Source: CAD feature listing. Evaluate the final solid. Frame: model axes, mm. Face numbers are marked on the shaded views. Round coordinates to 2 decimals unless told otherwise and drop trailing zeros. Write each question's results on one line, items separated by ' | '. Start each with the question number.
1. Draft query along Y for the marked faces 1 and 2. Return one class per face: released by +Y, released by -Y, zero draft, split by the parting line, or undercut.
2. Section A-A on y = 4.25. Give the number of separate pieces and of enclosed holes in the cut face, and give its area (3 significant figures).
3. Ray query, line 1 (X direction, y = 3.25, z = 0); line 2 (X direction, y = 1.75, z = 42) (3 decimals); line 3 (Z direction, x = 1, y = 11). Return the intervals inside material, ascending.
4. Contact query for flat-ended pins moving along their axis: pin 1 Ø6.5 at (y, z) = (9.5, 42.5) entering from +X; pin 2 Ø4 at (y, z) = (9, -42.5) entering from -X. Output: stop coordinate, or through.
from build123d import *

# Parameters (mm, degrees)
SKETCH1_W          = 304.8
SKETCH1_H          = 190.5
EXTRUDE1_DEPTH     = 12.7
SKETCH2_W          = 12.7
SKETCH2_H          = 19.05
EXTRUDE2_DEPTH     = 181.165514181
SKETCH3_R          = 1.5875
CUT_EXTRUDE1_DEPTH = 181.165514181
SKETCH4_R          = 2.032
CUT_EXTRUDE2_DEPTH = 181.165514181


with BuildPart() as part:
    # Sketch1 → Extrude1 (new body)
    with BuildSketch(Plane(origin=(0, 0, 0), x_dir=(1, 0, 0), z_dir=(0, 1, 0))):
        Rectangle(SKETCH1_W, SKETCH1_H)
    extrude(amount=EXTRUDE1_DEPTH)

    # Sketch2 → Extrude2 (cut, through all)
    with BuildSketch(Plane(origin=(0, 12.7, 0), x_dir=(1, 0, 0), z_dir=(0, 1, 0))):
        with Locations((-48.895, 44.45)):
            Rectangle(SKETCH2_W, SKETCH2_H)
        with Locations((48.895, 44.45)):
            Rectangle(SKETCH2_W, SKETCH2_H)
        with Locations((-48.895, -44.45)):
            Rectangle(SKETCH2_W, SKETCH2_H)
        with Locations((48.895, -44.45)):
            Rectangle(SKETCH2_W, SKETCH2_H)
        with Locations((146.05, 44.45)):
            Rectangle(SKETCH2_W, SKETCH2_H)
        with Locations((-146.05, 44.45)):
            Rectangle(SKETCH2_W, SKETCH2_H)
        with Locations((146.05, -44.45)):
            Rectangle(SKETCH2_W, SKETCH2_H)
        with Locations((-146.05, -44.45)):
            Rectangle(SKETCH2_W, SKETCH2_H)
    extrude(amount=-EXTRUDE2_DEPTH, mode=Mode.SUBTRACT)

    # Sketch3 → Cut-Extrude1 (cut, through all)
    with BuildSketch(Plane.XZ):
        with Locations(Location((50.8, 0, 0), (0, 0, 270))):
            Circle(SKETCH3_R)
        with Locations(Location((-50.8, 0, 0), (0, 0, 270))):
            Circle(SKETCH3_R)
    extrude(amount=-CUT_EXTRUDE1_DEPTH, mode=Mode.SUBTRACT)

    # Sketch4 → Cut-Extrude2 (cut, through all)
    with BuildSketch(Plane(origin=(0, 12.7, 0), x_dir=(1, 0, 0), z_dir=(0, 1, 0))):
        with Locations(Location((0, 22.225, 0), (0, 0, 270))):
            Circle(SKETCH4_R)
    extrude(amount=-CUT_EXTRUDE2_DEPTH, mode=Mode.SUBTRACT)


solid = part.part
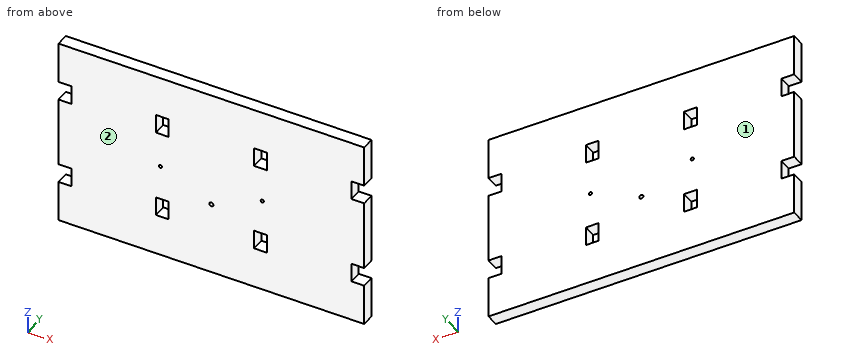
Taken from the geometry:
1) face 1: released by +Y | face 2: released by -Y
2) separate pieces: 1 | enclosed holes: 7 | area: 56,100 mm^2
3) line 1: -152.4 to -52.39, -49.21 to 49.21, 52.39 to 152.4 | line 2: -139.7 to -55.245, -42.545 to 42.545, 55.245 to 139.7 | line 3: -95.25 to -23.99, -20.46 to 95.25
4) pin 1: x = 139.7 | pin 2: x = -139.7
